The listing builds one solid part. Answer for the finished solid, in the listing's coordinates (mm). Round coordinates to 2 decimals unless told otherwise and drop trailing zeros. Write each loop counter-clockwise with the first axis right and the second up, starting at its lowest first coordinate (ties: lowest second). Pieces come first, ordered by that corner, then holes. Notation, with made-up numbers: (3.5, 0.5) - (50.5, 0.5) arc R6 cw to (50.5, 5.5) - close; hole circle Ø1 at (7, 36). An arc over 180 degrees is marked (long way). Answer as CSV lines item,"result". Start each with the question number.
Item 1: A cutting plane is placed at D-D on x = 12. Determine the outline of the cut face in (y, z), and give its area (3 significant figures).
Item 2: For a pull along X with two mould halves and no side action, classify faces 1 (the flat face through (15.24, 13.97, 1.16)), 2 (the cylindrical face through (22.013, -15.196, 1.165)), 3 (the flat face through (-28.719, -12.565, 1.165)) as pulls with the +X half, pulls with the -X half, needs draft (parallel to the pull), parting line crosses it, or undercut.
Item 3: Straight lines are drawn through the part: line 1 along Y through (x, z) = (0, 0.7); line 2 along X through (y, z) = (-15.5, 0.6); line 3 along Y through (x, z) = (6, 0.65). For each, find the intervals that lie inside material, in ascending order. Write a range as [from, to].
Item 4: A cutting plane is placed at B-B on x = -16.5. Determine the outline of the cut face in (y, z).
Item 5: A cutting plane is placed at C-C on z = 1.2. State how many separate pieces and enclosed holes the cut face has, and give its area (3 significant figures).
Item 6: A cutting plane is placed at A-A on y = 0. Determine the outline of the cut face in (x, z).
Item 7: A flat-ended cylindrical pin translates along its axis: pin 1 (2 mm diameter, centred on x = 6.02, y = -16, fed in from +Z). Find the tip coordinate at first contact, or state that the pin passes through.
```python
from build123d import *

# Parameters (mm, degrees)
F0_R     = 0.8001
F0_R_2   = 1.1811
F0_R_3   = 2.38125
F1_DEPTH = 2.3622


with BuildPart() as f1:
    # F0 (on Top) → F1 (new body)
    with BuildSketch(Plane.XY):
        with BuildLine():
            Line((-23.064947, -19.05), (0, -19.05))
            Line((0, -19.05), (23.064947, -19.05))
            Line((23.064947, -19.05), (34.217403, -6.259881))
            ThreePointArc((34.217403, -6.259881), (36.228268, 2.504018), (30.049558, 9.036479))
            Line((30.049558, 9.036479), (0, 19.05))
            Line((0, 19.05), (-30.049558, 9.036479))
            ThreePointArc((-30.049558, 9.036479), (-36.228268, 2.504018), (-34.217403, -6.259881))
            Line((-34.217403, -6.259881), (-23.064947, -19.05))
        make_face()
        with Locations((-22.1869, -14.4145)):
            Circle(F0_R, mode=Mode.SUBTRACT)
        with Locations((-6.016295, -16.003957)):
            Circle(F0_R_2, mode=Mode.SUBTRACT)
        with Locations((6.016295, -16.003957)):
            Circle(F0_R_2, mode=Mode.SUBTRACT)
        with Locations((0, -13.617562)):
            Circle(F0_R_2, mode=Mode.SUBTRACT)
        with Locations((22.1869, -14.4145)):
            Circle(F0_R, mode=Mode.SUBTRACT)
        with Locations((-28.5115, 0)):
            Circle(F0_R_3, mode=Mode.SUBTRACT)
        with Locations((-17.1069, 0)):
            Circle(F0_R_3, mode=Mode.SUBTRACT)
        with Locations((-5.7023, 0)):
            Circle(F0_R_3, mode=Mode.SUBTRACT)
        with Locations((5.7023, 0)):
            Circle(F0_R_3, mode=Mode.SUBTRACT)
        with Locations((17.1069, 0)):
            Circle(F0_R_3, mode=Mode.SUBTRACT)
        with Locations((28.5115, 0)):
            Circle(F0_R_3, mode=Mode.SUBTRACT)
        with Locations((0, 14.4145)):
            Circle(F0_R, mode=Mode.SUBTRACT)
    extrude(amount=F1_DEPTH)


solid = f1.part
```
Geometry says:
1,outline,"(-19.05, 0) - (15.05, 0) - (15.05, 2.36) - (-19.05, 2.36) - close"
1,area,"80.6 mm^2"
2,face 1,"pulls with the +X half"
2,face 2,"undercut"
2,face 3,"pulls with the -X half"
3,line 1,"y = [-19.05, -14.8], [-12.44, 13.61], [15.21, 19.05]"
3,line 2,"x = [-26.16, -7.08], [-4.95, 4.95], [7.08, 26.16]"
3,line 3,"y = [-19.05, -17.18], [-14.82, -2.36], [2.36, 17.05]"
4,outline,"(-19.05, 0) - (-2.3, 0) - (-2.3, 2.36) - (-19.05, 2.36) - close; (2.3, 0) - (13.55, 0) - (13.55, 2.36) - (2.3, 2.36) - close"
5,separate pieces,"1"
5,enclosed holes,"12"
5,area,"1,990 mm^2"
6,outline,"(-36.56, 0) - (-30.89, 0) - (-30.89, 2.36) - (-36.56, 2.36) - close; (-26.13, 0) - (-19.49, 0) - (-19.49, 2.36) - (-26.13, 2.36) - close; (-14.73, 0) - (-8.08, 0) - (-8.08, 2.36) - (-14.73, 2.36) - close; (-3.32, 0) - (3.32, 0) - (3.32, 2.36) - (-3.32, 2.36) - close; (8.08, 0) - (14.73, 0) - (14.73, 2.36) - (8.08, 2.36) - close; (19.49, 0) - (26.13, 0) - (26.13, 2.36) - (19.49, 2.36) - close; (30.89, 0) - (36.56, 0) - (36.56, 2.36) - (30.89, 2.36) - close"
7,pin 1,"passes through"
